```python
from build123d import *

# Parameters (mm, degrees)
SKETCH_1_W            = 100
SKETCH_1_H            = 100
EXTRUDE_1_DEPTH       = 100
SHELL_1_T             = -2
SHEET_START           = -51
SHEET_METAL_1_DEPTH   = 4.414213562
SHEET_START_2         = 46.585786438
SHEET_METAL_1_2_DEPTH = 4.414213562
SHEET_START_3         = -46.585786438
SHEET_METAL_1_3_DEPTH = 93.171572876
SHEET_METAL_1_4_DEPTH = 1.085786438
SHEET_START_4         = 45.5
SHEET_METAL_1_5_DEPTH = 1.085786438
SHEET_START_5         = -45.5
SHEET_METAL_1_6_DEPTH = 91
SHEET_METAL_1_7_DEPTH = 91
SHEET_METAL_1_8_DEPTH = 91


with BuildPart() as part:
    # Sketch 1 → 凸台-拉伸1 (new body)
    with BuildSketch(Plane(origin=(0, 0, 0), x_dir=(1, 0, 0), z_dir=(0, 1, 0))):
        Rectangle(SKETCH_1_W, SKETCH_1_H)
    extrude(amount=EXTRUDE_1_DEPTH)

    # 抽壳1
    shell_1_openings = [part.faces().sort_by_distance(p)[0] for p in [
        (0, 0, 0),
    ]]
    offset(amount=SHELL_1_T, openings=shell_1_openings, kind=Kind.INTERSECTION)

    # Sheet Metal 1: read off the stored shape, not the designer's step
    # Sheet Metal 1 outline → Sheet Metal 1 (cut)
    with BuildSketch(Plane.YZ.offset(SHEET_START)):
        Polygon((0, 50), (0, 46.585786438), (95.5, 46.585786438), (95.5, 45.5), (100, 45.5), (100, 50), align=None)
        Polygon((0, -46.585786438), (0, -50), (100, -50), (100, -45.5), (95.5, -45.5), (95.5, -46.585786438), align=None)
    extrude(amount=SHEET_METAL_1_DEPTH, mode=Mode.SUBTRACT)

    # Sheet Metal 1 2 outline → Sheet Metal 1 2 (cut)
    with BuildSketch(Plane.YZ.offset(SHEET_START_2)):
        Polygon((0, 50), (0, 46.585786438), (95.5, 46.585786438), (95.5, 45.5), (100, 45.5), (100, 50), align=None)
        Polygon((0, -46.585786438), (0, -50), (100, -50), (100, -45.5), (95.5, -45.5), (95.5, -46.585786438), align=None)
    extrude(amount=SHEET_METAL_1_2_DEPTH, mode=Mode.SUBTRACT)

    # Sheet Metal 1 3 outline → Sheet Metal 1 3 (cut)
    with BuildSketch(Plane.YZ.offset(SHEET_START_3)):
        with BuildLine():
            ThreePointArc((96, 50), (98.828427125, 48.828427125), (100, 46))
            Line((100, 46), (100, 50))
            Line((100, 50), (96, 50))
        make_face()
        with BuildLine():
            Line((100, -50), (100, -46))
            ThreePointArc((100, -46), (98.828427125, -48.828427125), (96, -50))
            Line((96, -50), (100, -50))
        make_face()
    extrude(amount=SHEET_METAL_1_3_DEPTH, mode=Mode.SUBTRACT)

    # Sheet Metal 1 4 outline → Sheet Metal 1 4 (cut)
    with BuildSketch(Plane.YZ.offset(SHEET_START_3)):
        with BuildLine():
            Line((98, 48), (98, 45.5))
            Line((98, 45.5), (100, 45.5))
            Line((100, 45.5), (100, 46))
            ThreePointArc((100, 46), (98.828427125, 48.828427125), (96, 50))
            Line((96, 50), (95.5, 50))
            Line((95.5, 50), (95.5, 48))
            Line((95.5, 48), (98, 48))
        make_face()
        with BuildLine():
            Line((100, -45.5), (98, -45.5))
            Line((98, -45.5), (98, -48))
            Line((98, -48), (95.5, -48))
            Line((95.5, -48), (95.5, -50))
            Line((95.5, -50), (96, -50))
            ThreePointArc((96, -50), (98.828427125, -48.828427125), (100, -46))
            Line((100, -46), (100, -45.5))
        make_face()
    extrude(amount=SHEET_METAL_1_4_DEPTH, mode=Mode.SUBTRACT)

    # Sheet Metal 1 5 outline → Sheet Metal 1 5 (cut)
    with BuildSketch(Plane.YZ.offset(SHEET_START_4)):
        with BuildLine():
            Line((98, 48), (98, 45.5))
            Line((98, 45.5), (100, 45.5))
            Line((100, 45.5), (100, 46))
            ThreePointArc((100, 46), (98.828427125, 48.828427125), (96, 50))
            Line((96, 50), (95.5, 50))
            Line((95.5, 50), (95.5, 48))
            Line((95.5, 48), (98, 48))
        make_face()
        with BuildLine():
            Line((100, -45.5), (98, -45.5))
            Line((98, -45.5), (98, -48))
            Line((98, -48), (95.5, -48))
            Line((95.5, -48), (95.5, -50))
            Line((95.5, -50), (96, -50))
            ThreePointArc((96, -50), (98.828427125, -48.828427125), (100, -46))
            Line((100, -46), (100, -45.5))
        make_face()
    extrude(amount=SHEET_METAL_1_5_DEPTH, mode=Mode.SUBTRACT)

    # Sheet Metal 1 6 outline → Sheet Metal 1 6 (add)
    with BuildSketch(Plane.YZ.offset(SHEET_START_5)):
        with BuildLine():
            ThreePointArc((96, 48), (97.414213562, 47.414213562), (98, 46))
            Line((98, 46), (98, 48))
            Line((98, 48), (96, 48))
        make_face()
        with BuildLine():
            Line((98, -48), (98, -46))
            ThreePointArc((98, -46), (97.414213562, -47.414213562), (96, -48))
            Line((96, -48), (98, -48))
        make_face()
    extrude(amount=SHEET_METAL_1_6_DEPTH)

    # Sheet Metal 1 7 outline → Sheet Metal 1 7 (cut)
    with BuildSketch(Plane.XY.offset(SHEET_START_5)):
        with BuildLine():
            Line((-50, 100), (-50, 96))
            ThreePointArc((-50, 96), (-48.828427125, 98.828427125), (-46, 100))
            Line((-46, 100), (-50, 100))
        make_face()
        with BuildLine():
            Line((50, 100), (46, 100))
            ThreePointArc((46, 100), (48.828427125, 98.828427125), (50, 96))
            Line((50, 96), (50, 100))
        make_face()
    extrude(amount=SHEET_METAL_1_7_DEPTH, mode=Mode.SUBTRACT)

    # Sheet Metal 1 8 outline → Sheet Metal 1 8 (add)
    with BuildSketch(Plane.XY.offset(SHEET_START_5)):
        with BuildLine():
            Line((-48, 98), (-48, 96))
            ThreePointArc((-48, 96), (-47.414213562, 97.414213562), (-46, 98))
            Line((-46, 98), (-48, 98))
        make_face()
        with BuildLine():
            Line((48, 98), (46, 98))
            ThreePointArc((46, 98), (47.414213562, 97.414213562), (48, 96))
            Line((48, 96), (48, 98))
        make_face()
    extrude(amount=SHEET_METAL_1_8_DEPTH)


solid = part.part
```
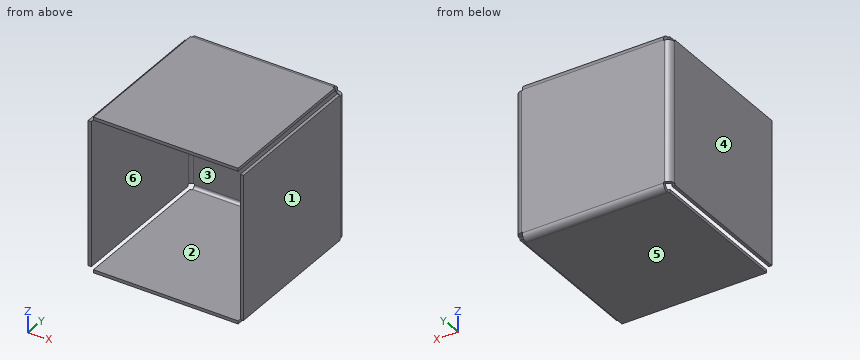
CAD build for the part. Positions are in the model's coordinates, mm. Face numbers are marked on the shaded views. A direction names the side the tool comes from. Coordinates: 2 decimals unless noted, no trailing zeros. Write each loop counter-clockwise with the first axis right and the second up, starting at its lowest first coordinate (ties: lowest second). Pieces come first, ordered by that corner, then holes. Notation, with made-up numbers: (27.5, 54) -> (54.5, 54) arc R24 cw to (54.5, 93) -> close; hole circle Ø3 at (-28, -11.75). An arc over 180 degrees is marked (long way). Return JSON: item names as keys, results as strings. Group by question number.
Q1. Flat gauge pins, fed straight in: pin 1 (4 mm diameter, centred on x = -39, z = 12, fed in from -Y); pin 2 (0.5 mm diameter, centred on x = 48.5, z = -46, fed in from +Y); pin 3 (3.5 mm diameter, centred on y = 98, z = 48.5, fed in from +X). Where does each tip first touch, or does it go through?
Q2. Cut at C-C, the plane x = 37. Give the cut face in (y, z), then the cut area to 3 significant figures.
Q3. Cut at B-B, the plane z = -5. Give the cut face in (x, y).
Q4. Drill centre lines: line 1 (X direction, y = 53.5, z = 15); line 2 (Y direction, x = -9, z = -3.5). Where is each one in solid material? Low to high.
Q5. Which spindle directions (+Z, -Z, +X, -X, +Y, -Y) get a long thin tool onto all of the face, cutting with end or side? Do the marked faces 1 and 2. Say none if no direction does.
Q6. Pull direction X, two halves, no side cores. Call the marked faces 3, 4, 5 and 6: released by +X, released by -X, zero draft, split by the parting line, or undercut.
Q7. Cut at A-A, the plane y = 58. Give the cut face in (x, z).
Returned:
{
 "1": {"pin 1": "stops at y = 98", "pin 2": "stops at y = 95.5", "pin 3": "stops at x = 45.5"},
 "2": {"outline": "(0, -50) -> (96, -50) arc R4 ccw to (100, -46) -> (100, 46) arc R4 ccw to (96, 50) -> (0, 50) -> (0, 48) -> (96, 48) arc R2 cw to (98, 46) -> (98, -46) arc R2 cw to (96, -48) -> (0, -48) -> close", "area": "587 mm2"},
 "3": {"outline": "(-50, 0) -> (-48, 0) -> (-48, 96) arc R2 cw to (-46, 98) -> (46, 98) arc R2 cw to (48, 96) -> (48, 0) -> (50, 0) -> (50, 96) arc R4 ccw to (46, 100) -> (-46, 100) arc R4 ccw to (-50, 96) -> close"},
 "4": {"line 1": "x = -50 to -48, 48 to 50", "line 2": "y = 98 to 100"},
 "5": {"face 1": "+Z, -Z, +X, +Y, -Y", "face 2": "+X, -X, -Y"},
 "6": {"face 3": "undercut", "face 4": "released by -X", "face 5": "zero draft", "face 6": "undercut"},
 "7": {"outline": "(-50, -46.59) -> (-48, -46.59) -> (-48, 46.59) -> (-50, 46.59) -> close; (-46.59, -50) -> (46.59, -50) -> (46.59, -48) -> (-46.59, -48) -> close; (-46.59, 48) -> (46.59, 48) -> (46.59, 50) -> (-46.59, 50) -> close; (48, -46.59) -> (50, -46.59) -> (50, 46.59) -> (48, 46.59) -> close"}
}
